from build123d import *

# Parameters (mm, degrees)
SKETCH1_R           = 9.5
SKETCH1_R_2         = 5.2
BOSS_EXTRUDE1_DEPTH = 29
SKETCH2_R           = 1.5
CUT_EXTRUDE1_DEPTH  = 30
CIRPATTERN1_COUNT   = 7
CHAMFER1_SIZE       = 1.5
CHAMFER1_SIZE2      = 1.050311307


with BuildPart() as part:
    # Sketch1 → Boss-Extrude1 (new body)
    with BuildSketch(Plane.XY):
        Circle(SKETCH1_R)
        Circle(SKETCH1_R_2, mode=Mode.SUBTRACT)
    extrude(amount=BOSS_EXTRUDE1_DEPTH)

    # Sketch2 → Cut-Extrude1 (cut, through all)
    with BuildSketch(Plane.XY.offset(29)):
        with Locations((0, 5.2)):
            Circle(SKETCH2_R)
    cut_extrude1 = extrude(amount=-CUT_EXTRUDE1_DEPTH, mode=Mode.SUBTRACT)

    # CirPattern1: Cut-Extrude1 ×7 about axis
    cirpattern1_axis = Axis((0, 0, 0), (0, 0, 1))
    for i in range(1, CIRPATTERN1_COUNT):
        add(cut_extrude1.rotate(cirpattern1_axis, i * 360 / CIRPATTERN1_COUNT), mode=Mode.SUBTRACT)

    # Chamfer1
    chamfer1_edges = [part.edges().sort_by_distance(p)[0] for p in [
        (-9.5, 0, 0),
        (-9.5, 0, 29),
    ]]
    chamfer1_side = [part.faces().sort_by_distance(p)[0] for p in [
        (-9.5, 0, 14.5),
    ]]
    chamfer(chamfer1_edges, length=CHAMFER1_SIZE, length2=CHAMFER1_SIZE2, reference=chamfer1_side[0])


solid = part.part
Check sheet for the modelled part. Datum: model origin and axes. Units: mm. A direction names the side the tool comes from. Round coordinates to 2 decimals unless told otherwise and drop trailing zeros. Order: outer loops, then holes, each group sorted by start corner. A loop starts at its lowest first (then second) coordinate and runs counter-clockwise, first axis right, second up.
Q1. Cross-section at A-A, the plane x = 0. Enter the section's corners in (y, z).
Filled sheet:
outline: (-9.5, 1.5) - (-8.45, 0) - (-5.2, 0) - (-5.2, 29) - (-8.45, 29) - (-9.5, 27.5) - close; (6.7, 0) - (8.45, 0) - (9.5, 1.5) - (9.5, 27.5) - (8.45, 29) - (6.7, 29) - close
Q2. Cross-section at B-B, the plane z = 6. Enter the section's corners in (x, y) (3 decimals), plus the area to 3 significant figures.
Filled sheet:
outline: circle Ø19 at (0, 0); hole (-5.189, 0.338) arc R1.5 ccw (long way) to (-4.528, -2.556) arc R5.2 ccw to (-3.5, -3.846) arc R1.5 ccw (long way) to (-0.825, -5.134) arc R5.2 ccw to (0.825, -5.134) arc R1.5 ccw (long way) to (3.5, -3.846) arc R5.2 ccw to (4.528, -2.556) arc R1.5 ccw (long way) to (5.189, 0.338) arc R5.2 ccw to (4.822, 1.947) arc R1.5 ccw (long way) to (2.971, 4.268) arc R5.2 ccw to (1.484, 4.984) arc R1.5 ccw (long way) to (-1.484, 4.984) arc R5.2 ccw to (-2.971, 4.268) arc R1.5 ccw (long way) to (-4.822, 1.947) arc R5.2 ccw to start
area: 172 mm2
Q3. Set-up check for faces 4 (the face through (-5.067, 1.168, 14.297)), 5 (the face through (-4, -4, 29)): record each of +Z, -Z, +X, -X, +Y, -Y from which the full face is reachable in a straight line by a thin tool's end or side.
Filled sheet:
face 4: +Z, -Z
face 5: +Z, +X, -X, +Y, -Y
Q4. Scan lines: L1, parallel to Y at x = 5.25, z = 3.25; L2, parallel to X at y = 5.2, z = 16.5; L3, parallel to Y at x = 3, z = 26.5. Record each from-to range of solid material in increasing order.
Filled sheet:
L1: y = -7.92 to -2.65, 0.33 to 2.32, 4.16 to 7.92
L2: x = -7.95 to -1.5, 1.5 to 7.95
L3: y = -9.01 to -5.99, 4.3 to 9.01
Q5. Cross-section at C-C, the plane y = 0. Enter the section's corners in (x, z).
Filled sheet:
outline: (-9.5, 1.5) - (-8.45, 0) - (-6.02, 0) - (-6.02, 29) - (-8.45, 29) - (-9.5, 27.5) - close; (6.02, 0) - (8.45, 0) - (9.5, 1.5) - (9.5, 27.5) - (8.45, 29) - (6.02, 29) - close
Q6. Depth check by flat-ended pin: P1, Ø2, axis at y = 6.5, z = 16.5, coming from the +X side; P2, Ø1, axis at y = -3, z = 13.5, coming from the +X side; P3, Ø3, axis at x = 3, z = 10.5, coming from the +Y side. Enter the tip coordinate at first touch or a pass-through.
Filled sheet:
P1: stops at x = 7.75
P2: stops at x = 9.17
P3: stops at y = 9.38
Q7. Draft check along X on faces 1 (the face through (4.38, -8.43, 14.32)), 2 (the face through (2.27, 4.68, 14.3)), 3 (the face through (-4, -4, 0)). Enter one of: pulls with the +X half, pulls with the -X half, needs draft (parallel to the pull), parting line crosses it, or undercut.
Filled sheet:
face 1: parting line crosses it
face 2: undercut
face 3: needs draft
